from build123d import *

# Parameters (mm, degrees)
CROQUIS1_W              = 330
CROQUIS1_H              = 135
SALIENTE_EXTRUIR1_DEPTH = 5
CROQUIS2_W              = 330
CROQUIS2_H              = 135
CROQUIS2_W_2            = 60
CROQUIS2_H_2            = 60
SALIENTE_EXTRUIR2_DEPTH = 30


with BuildPart() as part:
    # Croquis1 → Saliente-Extruir1 (new body)
    with BuildSketch(Plane(origin=(0, 0, 0), x_dir=(1, 0, 0), z_dir=(0, 1, 0))):
        Rectangle(CROQUIS1_W, CROQUIS1_H)
    extrude(amount=SALIENTE_EXTRUIR1_DEPTH)

    # Croquis2 → Saliente-Extruir2 (add)
    with BuildSketch(Plane(origin=(0, 5, 0), x_dir=(1, 0, 0), z_dir=(0, 1, 0))):
        Rectangle(CROQUIS2_W, CROQUIS2_H)
        with Locations((-130, 32.5)):
            Rectangle(CROQUIS2_W_2, CROQUIS2_H_2, mode=Mode.SUBTRACT)
        with Locations((-65, 32.5)):
            Rectangle(CROQUIS2_W_2, CROQUIS2_H_2, mode=Mode.SUBTRACT)
        with Locations((0, 32.5)):
            Rectangle(CROQUIS2_W_2, CROQUIS2_H_2, mode=Mode.SUBTRACT)
        with Locations((65, 32.5)):
            Rectangle(CROQUIS2_W_2, CROQUIS2_H_2, mode=Mode.SUBTRACT)
        with Locations((130, 32.5)):
            Rectangle(CROQUIS2_W_2, CROQUIS2_H_2, mode=Mode.SUBTRACT)
        with Locations((-130, -32.5)):
            Rectangle(CROQUIS2_W_2, CROQUIS2_H_2, mode=Mode.SUBTRACT)
        with Locations((-65, -32.5)):
            Rectangle(CROQUIS2_W_2, CROQUIS2_H_2, mode=Mode.SUBTRACT)
        with Locations((0, -32.5)):
            Rectangle(CROQUIS2_W_2, CROQUIS2_H_2, mode=Mode.SUBTRACT)
        with Locations((65, -32.5)):
            Rectangle(CROQUIS2_W_2, CROQUIS2_H_2, mode=Mode.SUBTRACT)
        with Locations((130, -32.5)):
            Rectangle(CROQUIS2_W_2, CROQUIS2_H_2, mode=Mode.SUBTRACT)
    extrude(amount=SALIENTE_EXTRUIR2_DEPTH)


solid = part.part
Verification items for the finished model (mm, model axes). Give positions to 0.01 mm unless a question says otherwise; leave off trailing zeros. Loops run counter-clockwise (first coordinate to the right, second up) from the corner with the lowest first, then second, coordinate; pieces in that order, holes last.
1) Depth check by flat-ended pin: pin 1 Ø4 at (x, z) = (46, 39) entering from +Y. Enter the tip coordinate at first touch or a pass-through.
2) Draft check along X on faces 1 (the flat face through (100, 20, -32)), 2 (the flat face through (-165, 17, 1)), 3 (the flat face through (-2, 17, 67.5)). Enter one of: pulls with the +X half, pulls with the -X half, needs draft (parallel to the pull), parting line crosses it, or undercut.
3) Thickness scan on line 1 along Z through (x, y) = (-4.5, 18.5); line 2 along X through (y, z) = (16, -53); line 3 along Y through (x, z) = (-114.5, 22). Record the ranges inside material, lowest first.
4) Sectioned sample at C-C, the plane y = 16.5. Count the separate pieces of the cut face and the enclosed holes in it, then the cut area to 3 significant figures.
5) Sectioned sample at B-B, the plane x = 54. Enter the section's corners in (y, z), then the cut area to 4 significant figures.
6) Sectioned sample at A-A, the plane z = 41.5. Enter the section's corners in (x, y), then the cut area to 3 significant figures.
Answers:
1. pin 1: stops at y = 5
2. face 1: undercut
2. face 2: pulls with the -X half
2. face 3: needs draft
3. line 1: z = -67.5 to -62.5, -2.5 to 2.5, 62.5 to 67.5
3. line 2: x = -165 to -160, -100 to -95, -35 to -30, 30 to 35, 95 to 100, 160 to 165
3. line 3: y = 0 to 5
4. separate pieces: 1
4. enclosed holes: 10
4. area: 8,550 mm2
5. outline: (0, -67.5) - (35, -67.5) - (35, -62.5) - (5, -62.5) - (5, -2.5) - (35, -2.5) - (35, 2.5) - (5, 2.5) - (5, 62.5) - (35, 62.5) - (35, 67.5) - (0, 67.5) - close
5. area: 1,125 mm2
6. outline: (-165, 0) - (165, 0) - (165, 35) - (160, 35) - (160, 5) - (100, 5) - (100, 35) - (95, 35) - (95, 5) - (35, 5) - (35, 35) - (30, 35) - (30, 5) - (-30, 5) - (-30, 35) - (-35, 35) - (-35, 5) - (-95, 5) - (-95, 35) - (-100, 35) - (-100, 5) - (-160, 5) - (-160, 35) - (-165, 35) - close
6. area: 2,550 mm2
